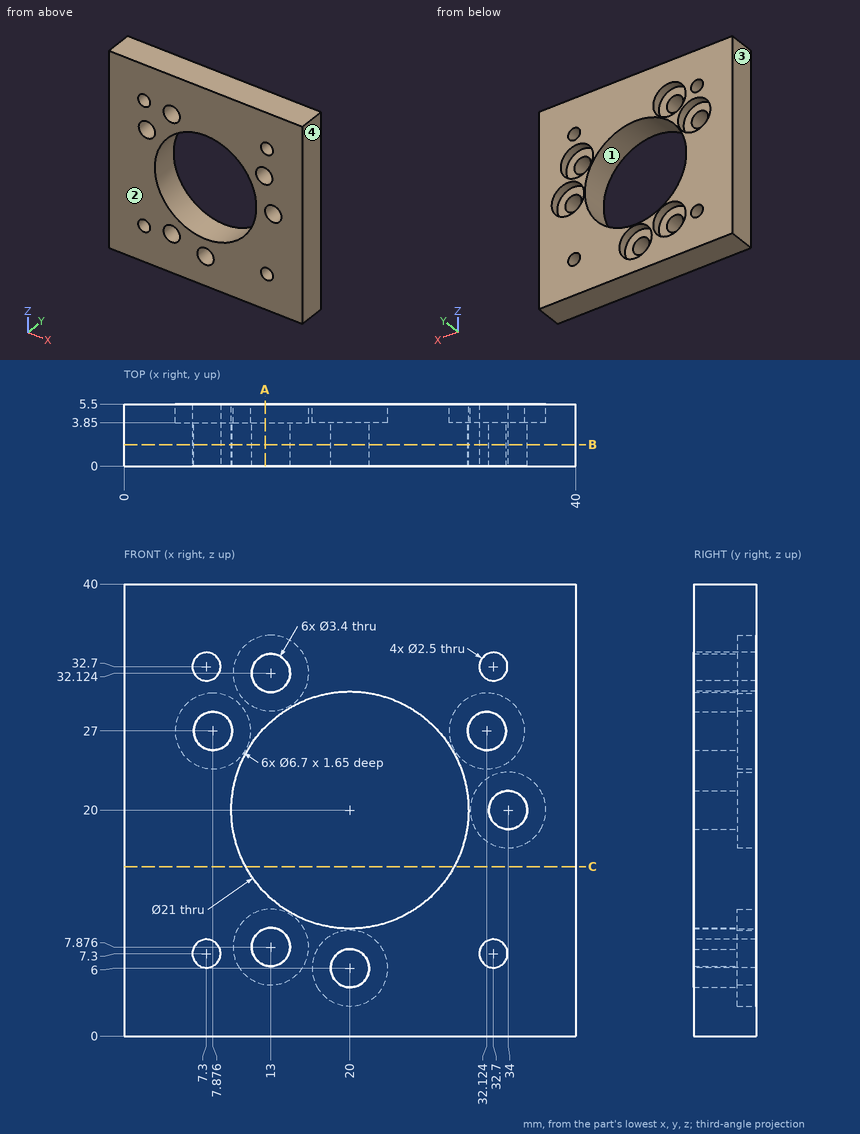
Print and shaded views of the part. All mm, measured from the part's lowest x, y and z. Give positions to 0.01 mm unless a question says otherwise; leave off trailing zeros. Loops run counter-clockwise (first coordinate to the right, second up) from the corner with the lowest first, then second, coordinate; pieces in that order, holes last. Notation, with made-up numbers: (48.5, 66) -> (81.5, 66) arc R17 cw to (81.5, 95) -> close; hole circle Ø7 at (19.25, -7). An arc over 180 degrees is marked (long way). Use a Markdown table: item, result.
1. Slice it at C-C (z = 15). List the corners of the cut face in (x, y).
Check result:
| item | result |
|---|---|
| outline | (0, 0) -> (10.77, 0) -> (10.77, 5.5) -> (0, 5.5) -> close; (29.23, 0) -> (40, 0) -> (40, 5.5) -> (29.23, 5.5) -> close |
2. Slice it at A-A (x = 12.5). List the corners of the cut face in (y, z).
Check result:
| item | result |
|---|---|
| outline | (0, 0) -> (5.5, 0) -> (5.5, 4.56) -> (3.85, 4.56) -> (3.85, 6.25) -> (0, 6.25) -> close; (0, 9.5) -> (3.85, 9.5) -> (3.85, 11.19) -> (5.5, 11.19) -> (5.5, 12.65) -> (0, 12.65) -> close; (0, 27.35) -> (5.5, 27.35) -> (5.5, 28.81) -> (3.85, 28.81) -> (3.85, 30.5) -> (0, 30.5) -> close; (0, 33.75) -> (3.85, 33.75) -> (3.85, 35.44) -> (5.5, 35.44) -> (5.5, 40) -> (0, 40) -> close |
3. Slice it at B-B (y = 1.9). Give the number of separate pieces and of enclosed holes in the cut face, plus the area to 3 significant figures.
Check result:
| item | result |
|---|---|
| separate pieces | 1 |
| enclosed holes | 11 |
| area | 1,180 mm^2 |
4. Flat gauge pins, fed straight in: pin 1 (1.5 mm diameter, centred on x = 32.7, z = 32.7, fed in from +Y); pin 2 (4 mm diameter, centred on x = 13, z = 32.12, fed in from +Y). Where does each tip first touch, or does it go through?
Check result:
| item | result |
|---|---|
| pin 1 | passes through |
| pin 2 | stops at y = 3.85 |
5. Wall check: L1, parallel to X at y = 5.1, z = 20; L2, parallel to X at y = 3.95, z = 24 (1 decimal); L3, parallel to X at y = 4.9, z = 27 (1 decimal). Give the ranges that are in metal, low to high. Write a range as [from, to].
Check result:
| item | result |
|---|---|
| L1 | x = [0, 9.5], [30.5, 30.65], [37.35, 40] |
| L2 | x = [0, 6.4], [9.4, 10.3], [29.7, 30.6], [33.6, 40] |
| L3 | x = [0, 4.5], [11.2, 12.2], [27.8, 28.8], [35.5, 40] |
6. Mould opens along X. For the marked faces 1, 2, 3 and 4 say: pulls with the +X half, pulls with the -X half, needs draft (parallel to the pull), parting line crosses it, or undercut.
Check result:
| item | result |
|---|---|
| face 1 | undercut |
| face 2 | needs draft |
| face 3 | pulls with the -X half |
| face 4 | pulls with the +X half |
